Autodesk Inventor part; units mm, degrees
ref_plane "YZ Plane" through (0, 0, 0) normal (1, 0, 0) x (0, 1, 0)
ref_plane "XZ Plane" through (0, 0, 0) normal (0, 1, 0) x (-1, 0, 0)
ref_plane "XY Plane" through (0, 0, 0) normal (0, 0, 1) x (1, 0, 0)
sketch "Skizze1" plane through (0, 0, 0) normal (0, 1, 0) x (-1, 0, 0)
  line L0 (0, 0) -> (5, 0)
  line L1 (5, 0) -> (5, -180)
  line L2 (5, -180) -> (0, -180)
  line L3 (0, -180) -> (0, 0)
  dimension "d0" = 180
  dimension "d1" = 10
revolve "Umdrehung1" add sketch "Skizze1" angle 360 about axis through (0, 0, -180) along (0, 0, 1)
thread "Gewinde1"
chamfer "Fase1" distance 2 angle 45 1 edges at (5, 0, 0)
mirror "Spiegeln1" about plane through (0, 0, -180) normal (0, 0, -1)
properties part number "Gewindestange_360" material "Stahl AISI 4130"
The model under review builds one solid part; all positions refer to its coordinate system, in mm. Coordinates: 2 decimals unless noted, no trailing zeros. Write each loop counter-clockwise with the first axis right and the second up, starting at its lowest first coordinate (ties: lowest second). Pieces come first, ordered by that corner, then holes. Notation, with made-up numbers: (28.25, 54.5) - (35.25, 54.5) arc R24 ccw to (35.25, 65.5) - close; hole circle Ø4 at (-2, -7). An arc over 180 degrees is marked (long way). Answer in a Markdown table with one row per item. Add a question column.
Q1. Consider section A-A on z = -319.5. Give the boundary of the cut face in (x, y).
Q2. Clearance check with flat-ended pins moving along their axes: pin 1 (2 mm diameter, centred on x = -2.5, z = -311.5, fed in from -Y); pin 2 (1 mm diameter, centred on x = -3, z = -196, fed in from -Y); pin 3 (1 mm diameter, centred on x = 2.5, z = -151.5, fed in from -Y). State where each tip first meets the part, or that it passes through.
Q3. To check wall thickness, follow line 1 along X through (y, z) = (-4, -210); line 2 along Z through (x, y) = (-0.5, -3); line 3 along X through (y, z) = (-0.25, -283). State the ranges of each line that lie inside material, in increasing order. Write a range as from..to.
Answers below:
| question | item | result |
|---|---|---|
| 1 | outline | circle Ø10 at (0, 0) |
| 2 | pin 1 | y = -4.77 |
| 2 | pin 2 | y = -4.33 |
| 2 | pin 3 | y = -4.58 |
| 3 | line 1 | -3..3 |
| 3 | line 2 | -359.96..-0.04 |
| 3 | line 3 | -4.99..4.99 |
